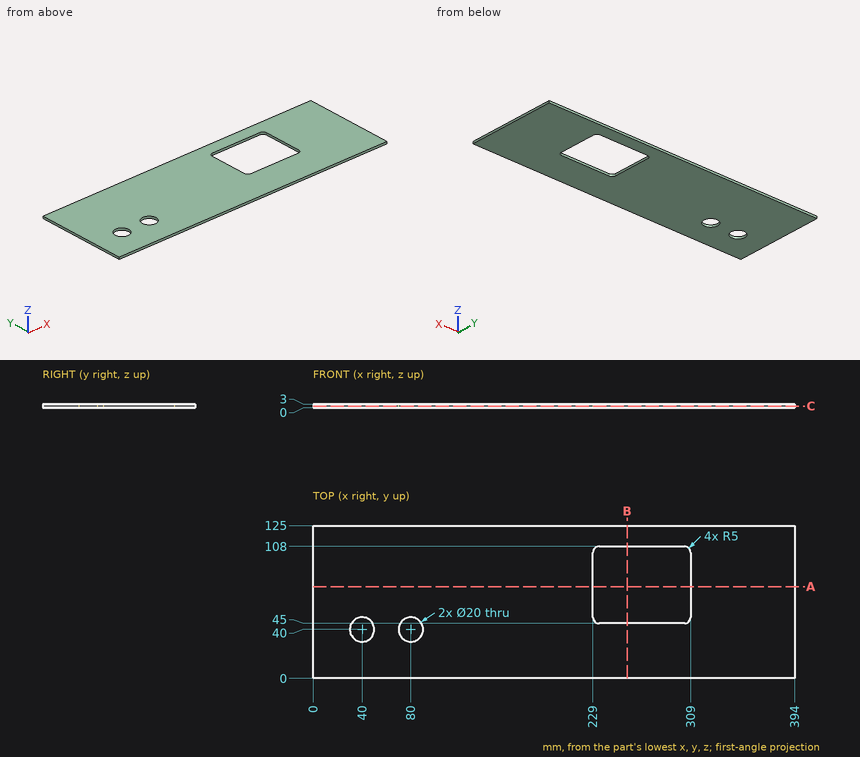
Drawing for the job (mm, zero at the part's lowest x, y, z). Give positions to 0.01 mm unless a question says otherwise; leave off trailing zeros. Loops run counter-clockwise (first coordinate to the right, second up) from the corner with the lowest first, then second, coordinate; pieces in that order, holes last.
(1) Band-saw the part on B-B (x = 257). Write the cut outline in (y, z).
Return value:
outline: (0, 0) - (45, 0) - (45, 3) - (0, 3) - close; (108, 0) - (125, 0) - (125, 3) - (108, 3) - close
(2) Pin check, flat tip, straight feed: pin 1 (18 mm diameter, centred on x = 40, y = 40, fed in from +Z). Stop position of the tip, or through.
Return value:
pin 1: passes through
(3) Band-saw the part on C-C (z = 1.3). Write the cut outline in (x, y), and give its area (3 significant figures).
Return value:
outline: (0, 0) - (394, 0) - (394, 125) - (0, 125) - close; hole circle Ø20 at (40, 40); hole circle Ø20 at (80, 40); hole (229, 50) arc R5 ccw to (234, 45) - (304, 45) arc R5 ccw to (309, 50) - (309, 103) arc R5 ccw to (304, 108) - (234, 108) arc R5 ccw to (229, 103) - close
area: 43,600 mm2
(4) Drill centre lines: line 1 along Y through (x, z) = (271.5, 2.7); line 2 along X through (y, z) = (49, 2.3); line 3 along X through (y, z) = (67.5, 2.3). Where is each one in solid material? Low to high.
Return value:
line 1: y = 0 to 45, 108 to 125
line 2: x = 0 to 35.64, 44.36 to 75.64, 84.36 to 229.1, 308.9 to 394
line 3: x = 0 to 229, 309 to 394
(5) Band-saw the part on A-A (y = 75). Write the cut outline in (x, z), and give its area (3 significant figures).
Return value:
outline: (0, 0) - (229, 0) - (229, 3) - (0, 3) - close; (309, 0) - (394, 0) - (394, 3) - (309, 3) - close
area: 942 mm2
